from build123d import *

# Parameters (mm, degrees)
SKETCH_1_W          = 250
SKETCH_1_H          = 170
SKETCH_1_R          = 3
EXTRUDE_1_DEPTH     = 3
FILLET_1_R          = 15
SKETCH_2_R          = 1.5
SKETCH_2_R_2        = 13.5
CUT_EXTRUDE_1_DEPTH = 152.191931002


with BuildPart() as part:
    # 草图1 → 凸台-拉伸1 (new body)
    with BuildSketch(Plane(origin=(0, 0, 0), x_dir=(1, 0, 0), z_dir=(0, 1, 0))):
        Rectangle(SKETCH_1_W, SKETCH_1_H)
        with Locations(Location((-105, 75, 0), (0, 0, 270))):
            Circle(SKETCH_1_R, mode=Mode.SUBTRACT)
        with Locations(Location((105, 75, 0), (0, 0, 270))):
            Circle(SKETCH_1_R, mode=Mode.SUBTRACT)
        with Locations(Location((-105, -75, 0), (0, 0, 270))):
            Circle(SKETCH_1_R, mode=Mode.SUBTRACT)
        with Locations(Location((105, -75, 0), (0, 0, 270))):
            Circle(SKETCH_1_R, mode=Mode.SUBTRACT)
    extrude(amount=EXTRUDE_1_DEPTH)

    # 圆角1
    fillet_1_edges = [part.edges().sort_by_distance(p)[0] for p in [
        (125, 1.5, 85),
        (-125, 1.5, 85),
        (-125, 1.5, -85),
        (125, 1.5, -85),
    ]]
    fillet(fillet_1_edges, radius=FILLET_1_R)

    # 草图2 → 切除-拉伸1 (cut, through all)
    with BuildSketch(Plane(origin=(0, 0, 0), x_dir=(1, 0, 0), z_dir=(0, 1, 0))):
        with Locations(Location((0, 21, 0), (0, 0, 270))):
            Circle(SKETCH_2_R)
        with Locations(Location((18.186533479, 10.5, 0), (0, 0, 270))):
            Circle(SKETCH_2_R)
        with Locations(Location((18.186533479, -10.5, 0), (0, 0, 270))):
            Circle(SKETCH_2_R)
        with Locations(Location((0, -21, 0), (0, 0, 270))):
            Circle(SKETCH_2_R)
        with Locations(Location((-18.186533479, -10.5, 0), (0, 0, 270))):
            Circle(SKETCH_2_R)
        with Locations(Location((-18.186533479, 10.5, 0), (0, 0, 270))):
            Circle(SKETCH_2_R)
        with Locations(Location((31, 0, 0), (0, 0, 270))):
            Circle(SKETCH_2_R)
        with Locations(Location((15.5, -26.846787517, 0), (0, 0, 270))):
            Circle(SKETCH_2_R)
        with Locations(Location((-15.5, -26.846787517, 0), (0, 0, 270))):
            Circle(SKETCH_2_R)
        with Locations(Location((-31, 0, 0), (0, 0, 270))):
            Circle(SKETCH_2_R)
        with Locations(Location((-15.5, 26.846787517, 0), (0, 0, 270))):
            Circle(SKETCH_2_R)
        with Locations(Location((15.5, 26.846787517, 0), (0, 0, 270))):
            Circle(SKETCH_2_R)
        with Locations(Location((0, 0, 0), (0, 0, 270))):
            Circle(SKETCH_2_R_2)
    extrude(amount=CUT_EXTRUDE_1_DEPTH, mode=Mode.SUBTRACT)


solid = part.part
Input: part model. Units: mm. Frame: model coordinates. Give positions to 0.01 mm unless a question says otherwise; leave off trailing zeros. Order: outer loops, then holes, each group sorted by start corner. A loop starts at its lowest first (then second) coordinate and runs counter-clockwise, first axis right, second up. Notation, with made-up numbers: M 47,7.25 L 66,7.25 A5 cw 66,11.25 Z; hole C 22,78.5 d5. An arc over 180 degrees is marked long. Answer as a JSON object with one key per item and string values.
1. Cut plane B-B, the plane z = 75. Output: boundary loops of the cut face in (x, y), and give its area (3 significant figures).
Result sheet:
{"outline": "M -124.14,0 L -108,0 L -108,3 L -124.14,3 Z; M -102,0 L 102,0 L 102,3 L -102,3 Z; M 108,0 L 124.14,0 L 124.14,3 L 108,3 Z", "area": "709 mm²"}
2. Pull-direction query (X, two-part tool) for faces 1 (the cylindrical face through (103.2, 1.5, 72.6)), 2 (the flat face through (-2, 3, -20)), 3 (the cylindrical face through (120.49, 1.52, -80.72)); classes: +X half, -X half, draft (parallel to the pull), parting line (faces both ways), or undercut.
Result sheet:
{"face 1": "undercut", "face 2": "draft", "face 3": "+X half"}
3. First-contact query: P1, Ø8, axis at x = 105, z = 75, coming from the +Y side; P2, Ø1.8, axis at x = -15.5, z = -26.85, coming from the -Y side. Flat tips, straight axial feed; report the tip coordinate or a pass-through.
Result sheet:
{"P1": "y = 3", "P2": "through"}
4. Ray query, line 1 (Z direction, x = 0, y = 2.05); line 2 (X direction, y = 0.75, z = 0); line 3 (Z direction, x = 15.5, y = 1). Return the intervals inside material, ascending. Write a range as [from, to].
Result sheet:
{"line 1": "[-85, -22.5], [-19.5, -13.5], [13.5, 19.5], [22.5, 85]", "line 2": "[-125, -32.5], [-29.5, -13.5], [13.5, 29.5], [32.5, 125]", "line 3": "[-85, -28.35], [-25.35, 25.35], [28.35, 85]"}
5. Cut plane A-A, the plane x = -105. Output: boundary loops of the cut face in (y, z).
Result sheet:
{"outline": "M 0,-85 L 3,-85 L 3,-78 L 0,-78 Z; M 0,-72 L 3,-72 L 3,72 L 0,72 Z; M 0,78 L 3,78 L 3,85 L 0,85 Z"}
6. Cut plane C-C, the plane y = 2.5. State how many separate pieces and enclosed holes the cut face has, and give its area (3 significant figures).
Result sheet:
{"separate pieces": "1", "enclosed holes": "17", "area": "41,500 mm²"}
